```python
from build123d import *

# Parameters (mm, degrees)
ESQUISSE1_R        = 15.25
ESQUISSE1_R_2      = 1.85
ESQUISSE1_R_3      = 2
ESQUISSE1_R_4      = 1
BOSS_EXTRU_1_DEPTH = 1


with BuildPart() as part:
    # Esquisse1 → Boss.-Extru.1 (new body)
    with BuildSketch(Plane.XY):
        with BuildLine():
            Line((37.808765603, 14.517136205), (14.517136205, 37.808765603))
            ThreePointArc((14.517136205, 37.808765603), (0, 40.5), (-14.517136205, 37.808765603))
            Line((-14.517136205, 37.808765603), (-37.808765603, 14.517136205))
            ThreePointArc((-37.808765603, 14.517136205), (-40.5, 0), (-37.808765603, -14.517136205))
            Line((-37.808765603, -14.517136205), (-14.517136205, -37.808765603))
            ThreePointArc((-14.517136205, -37.808765603), (0, -40.5), (14.517136205, -37.808765603))
            Line((14.517136205, -37.808765603), (37.808765603, -14.517136205))
            ThreePointArc((37.808765603, -14.517136205), (40.5, 0), (37.808765603, 14.517136205))
        make_face()
        Circle(ESQUISSE1_R, mode=Mode.SUBTRACT)
        with Locations((21.566756826, 21.566756826)):
            Circle(ESQUISSE1_R_2, mode=Mode.SUBTRACT)
        with Locations(Location((-21.566756826, -21.566756826, 0), (0, 0, 180))):
            Circle(ESQUISSE1_R_2, mode=Mode.SUBTRACT)
        with Locations((-21.566756826, 21.566756826)):
            Circle(ESQUISSE1_R_2, mode=Mode.SUBTRACT)
        with Locations(Location((21.566756826, -21.566756826, 0), (0, 0, 180))):
            Circle(ESQUISSE1_R_2, mode=Mode.SUBTRACT)
        with Locations((-12.727922061, 18.384776311)):
            Circle(ESQUISSE1_R_3, mode=Mode.SUBTRACT)
        with Locations(Location((-18.384776311, 12.727922061, 0), (0, 0, 180))):
            Circle(ESQUISSE1_R_3, mode=Mode.SUBTRACT)
        with Locations((12.727922061, -18.384776311)):
            Circle(ESQUISSE1_R_3, mode=Mode.SUBTRACT)
        with Locations(Location((18.384776311, -12.727922061, 0), (0, 0, 180))):
            Circle(ESQUISSE1_R_3, mode=Mode.SUBTRACT)
        with Locations((19, -3.35)):
            Circle(ESQUISSE1_R_4, mode=Mode.SUBTRACT)
        with Locations((32, -3.35)):
            Circle(ESQUISSE1_R_4, mode=Mode.SUBTRACT)
        with Locations(Location((32, 3.35, 0), (0, 0, 180))):
            Circle(ESQUISSE1_R_4, mode=Mode.SUBTRACT)
        with Locations(Location((19, 3.35, 0), (0, 0, 180))):
            Circle(ESQUISSE1_R_4, mode=Mode.SUBTRACT)
        with Locations(Location((-19, -3.35, 0), (0, 0, 180))):
            Circle(ESQUISSE1_R_4, mode=Mode.SUBTRACT)
        with Locations(Location((-32, -3.35, 0), (0, 0, 180))):
            Circle(ESQUISSE1_R_4, mode=Mode.SUBTRACT)
        with Locations((-32, 3.35)):
            Circle(ESQUISSE1_R_4, mode=Mode.SUBTRACT)
        with Locations((-19, 3.35)):
            Circle(ESQUISSE1_R_4, mode=Mode.SUBTRACT)
        with Locations((3.35, 19)):
            Circle(ESQUISSE1_R_4, mode=Mode.SUBTRACT)
        with Locations((3.35, 32)):
            Circle(ESQUISSE1_R_4, mode=Mode.SUBTRACT)
        with Locations(Location((-3.35, 32, 0), (0, 0, 180))):
            Circle(ESQUISSE1_R_4, mode=Mode.SUBTRACT)
        with Locations(Location((-3.35, 19, 0), (0, 0, 180))):
            Circle(ESQUISSE1_R_4, mode=Mode.SUBTRACT)
        with Locations(Location((3.35, -19, 0), (0, 0, 180))):
            Circle(ESQUISSE1_R_4, mode=Mode.SUBTRACT)
        with Locations(Location((3.35, -32, 0), (0, 0, 180))):
            Circle(ESQUISSE1_R_4, mode=Mode.SUBTRACT)
        with Locations((-3.35, -32)):
            Circle(ESQUISSE1_R_4, mode=Mode.SUBTRACT)
        with Locations((-3.35, -19)):
            Circle(ESQUISSE1_R_4, mode=Mode.SUBTRACT)
    extrude(amount=BOSS_EXTRU_1_DEPTH)


solid = part.part
```
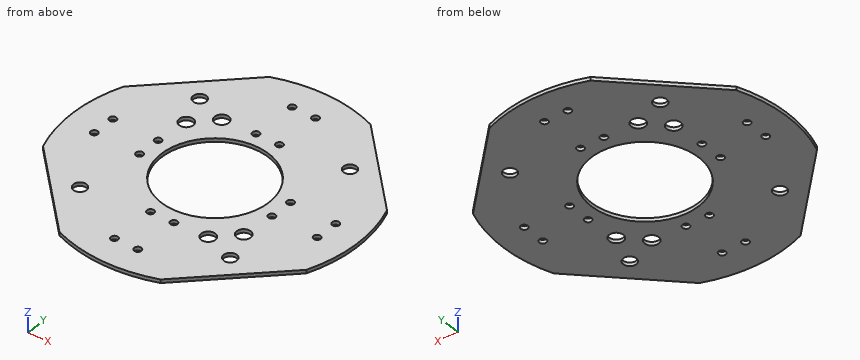
Part model, mm, in its own coordinate system. Coordinates: 2 decimals unless noted, no trailing zeros. Write each loop counter-clockwise with the first axis right and the second up, starting at its lowest first coordinate (ties: lowest second). Pieces come first, ordered by that corner, then holes.
Item 1: Slice it at B-B (y = -3.35). Write the cut outline in (x, z).
Item 2: Slice it at C-C (z = 0.4). Count the separate pieces of the cut face and the enclosed holes in it, and give its area (3 significant figures).
Item 3: Slice it at A-A (x = 0). Write the cut outline in (y, z), and give its area (3 significant figures).
Item 4: Probe line 1 (Y direction, x = 32, z = 0.45); line 2 (Y direction, x = 23, z = 0.35); line 3 (X direction, y = -22, z = 0.65). List the from-to ranges inside material, lowest first.
Item 5: Slice it at D-D (x = 32). Write the cut outline in (y, z), and give its area (3 significant figures).
Results found:
1. outline: (-40.36, 0) - (-33, 0) - (-33, 1) - (-40.36, 1) - close; (-31, 0) - (-20, 0) - (-20, 1) - (-31, 1) - close; (-18, 0) - (-14.88, 0) - (-14.88, 1) - (-18, 1) - close; (14.88, 0) - (18, 0) - (18, 1) - (14.88, 1) - close; (20, 0) - (31, 0) - (31, 1) - (20, 1) - close; (33, 0) - (40.36, 0) - (40.36, 1) - (33, 1) - close
2. separate pieces: 1
2. enclosed holes: 25
2. area: 3,970 mm2
3. outline: (-40.5, 0) - (-15.25, 0) - (-15.25, 1) - (-40.5, 1) - close; (15.25, 0) - (40.5, 0) - (40.5, 1) - (15.25, 1) - close
3. area: 50.5 mm2
4. line 1: y = -20.33 to -4.35, -2.35 to 2.35, 4.35 to 20.33
4. line 2: y = -29.33 to -22.74, -20.4 to 20.4, 22.74 to 29.33
4. line 3: x = -30.33 to -23.37, -19.77 to 19.77, 23.37 to 30.33
5. outline: (-20.33, 0) - (-4.35, 0) - (-4.35, 1) - (-20.33, 1) - close; (-2.35, 0) - (2.35, 0) - (2.35, 1) - (-2.35, 1) - close; (4.35, 0) - (20.33, 0) - (20.33, 1) - (4.35, 1) - close
5. area: 36.7 mm2
